CAD build for the part. Positions are in the model's coordinates, mm. A direction names the side the tool comes from. Give positions to 0.01 mm unless a question says otherwise; leave off trailing zeros. Loops run counter-clockwise (first coordinate to the right, second up) from the corner with the lowest first, then second, coordinate; pieces in that order, holes last.
Item 1: Which spindle directions (+Z, -Z, +X, -X, +Y, -Y) get a long thin tool onto all of the face, cutting with end or side? Do faces 4 (the flat face through (24, 0, -7)), 5 (the flat face through (21.5, 0, -7)), 6 (the cylindrical face through (-176.276, 226.457, 13.151)), 7 (the flat face through (226, 208, 12)). Say none if no direction does.
Item 2: Drop flat-ended pins along their axis: P1, Ø4, axis at x = -89.5, y = 148.5, coming from the -Z side; P2, Ø16.5, axis at y = 5.5, z = -9.5, coming from the -X side; P3, Ø4.5, axis at y = -1, z = -8, coming from the +X side. Give the stop position or say it passes through.
Item 3: Saw through at B-B on y = 180.5. Give the cut face in (x, z), plus the area to 3 significant figures.
Item 4: Probe probe 1 along Z at (x, y) = (-43, -23); probe 2 along Y at (x, z) = (216, 9). List the from-to ranges inside material, lowest first.
Item 5: Saw through at A-A on x = -140. Give the cut face in (y, z).
Item 6: Mould opens along Y. For faces 1 (the flat face through (0, -10, -7)), 2 (the flat face through (0, -12.5, -7)), 3 (the flat face through (22, -49, 0)) say: released by +Y, released by -Y, zero draft, split by the parting line, or undercut.
Autodesk Inventor part; units mm, degrees
ref_plane "YZ Plane" through (0, 0, 0) normal (1, 0, 0) x (0, 1, 0)
ref_plane "XZ Plane" through (0, 0, 0) normal (0, 1, 0) x (-1, 0, 0)
ref_plane "XY Plane" through (0, 0, 0) normal (0, 0, 1) x (1, 0, 0)
sketch "Boceto1" plane through (0, 0, 0) normal (0, 0, 1) x (1, 0, 0)
  line L0 (-160.5, 235) -> (210.5, 235)
  line L1 (242.5, 208) -> (242.5, -230)
  line L2 (237.5, -235) -> (-187.5, -235)
  line L3 (-192.5, -230) -> (-192.5, 208)
  line L4 (-160.5, 235) -> (-160.5, 208)
  line L5 (-160.5, 208) -> (-192.5, 208)
  line L6 (210.5, 235) -> (210.5, 208)
  line L7 (210.5, 208) -> (242.5, 208)
  arc A0 (-192.5, -230) -> (-187.5, -235) centre (-187.5, -230) ccw
  arc A1 (237.5, -235) -> (242.5, -230) centre (237.5, -230) ccw
  point P0 (0, 0)
  point P1 (242.5, -235)
  point P2 (-192.5, -235)
  dimension "d0" = 435
  dimension "d2" = 32
  dimension "d3" = 27
  dimension "d4" = 32
  dimension "d18" = 5
extrude "Extrusión1" add sketch "Boceto1" along normal blind 25
sketch "Boceto2" plane through (210.5, 208, 0) normal (1, 0, 0) x (0, 0, -1)
  line L0 (0, 0) -> (-25, 0)
  circle A0 centre (-12.5, 13.5) radius 5
  point P0 (0, -208)
  dimension "d7" = 10
extrude "Extrusión2" add sketch "Boceto2" along normal blind 32 and the other way blind 403
sketch "Boceto3" plane through (0, 0, 0) normal (0, 0, -1) x (-1, 0, 0)
  line L0 (-21.5, 10) -> (21.5, 10)
  line L1 (21.5, 10) -> (21.5, -10)
  line L2 (21.5, -10) -> (-21.5, -10)
  line L3 (-21.5, -10) -> (-21.5, 10)
  line L4 (-21.5, 10) -> (21.5, -10) construction
  line L5 (21.5, 10) -> (-21.5, -10) construction
  line L6 (24, 12.5) -> (-24, 12.5)
  line L7 (-24, 12.5) -> (-24, -12.5)
  line L8 (-24, -12.5) -> (24, -12.5)
  line L9 (24, -12.5) -> (24, 12.5)
  line L10 (24, 12.5) -> (-24, -12.5) construction
  line L11 (-24, 12.5) -> (24, -12.5) construction
  point P0 (0, 0)
  dimension "d14" = 48
  dimension "d15" = 25
extrude "Extrusión3" add sketch "Boceto3" along normal blind 15
properties part number "tapa"
Results below:
1. face 4: -Z, +X, +Y, -Y
1. face 5: -Z
1. face 6: -X
1. face 7: +Z, -Z, +X
2. P1: stops at z = 0
2. P2: stops at x = -24
2. P3: stops at x = 24
3. outline: (-192.5, 0) - (242.5, 0) - (242.5, 25) - (-192.5, 25) - close
3. area: 10,900 mm2
4. probe 1: z = 0 to 25
4. probe 2: y = -235 to 208, 217.93 to 225.07
5. outline: (-235, 0) - (235, 0) - (235, 25) - (-235, 25) - close
6. face 1: undercut
6. face 2: released by -Y
6. face 3: zero draft
